Read the model definition and answer for the solid it produces. Units are mm, in the model's axes. A direction names the side the tool comes from. Coordinates: 2 decimals unless noted, no trailing zeros. Order: outer loops, then holes, each group sorted by start corner. A loop starts at its lowest first (then second) coordinate and runs counter-clockwise, first axis right, second up. Notation, with made-up numbers: (46, -19.75) -> (96, -19.75) arc R30 ccw to (96, 13.25) -> close; hole circle Ø9 at (66.5, 72). An arc over 180 degrees is marked (long way). Use CSV: the item, a comma, the result in double quotes.
```python
from build123d import *

# Parameters (mm, degrees)
SKETCH1_R           = 2.75
SKETCH1_R_2         = 1.475
BOSS_EXTRUDE1_DEPTH = 31.95
BOSS_EXTRUDE2_START = -31.95
BOSS_EXTRUDE2_DEPTH = 31.95
SKETCH3_R           = 1.475
BOSS_EXTRUDE3_DEPTH = 31.95
SKETCH4_R           = 1.475
CUT_EXTRUDE1_DEPTH  = 10
CUT_EXTRUDE2_START  = -10
SKETCH5_R           = 1.475
CUT_EXTRUDE2_DEPTH  = 10


with BuildPart() as part:
    # Sketch1 → Boss-Extrude1 (new body)
    with BuildSketch(Plane.XY):
        Circle(SKETCH1_R)
        Circle(SKETCH1_R_2, mode=Mode.SUBTRACT)
    extrude(amount=BOSS_EXTRUDE1_DEPTH)

    # Sketch2 → Boss-Extrude2 (add)
    with BuildSketch(Plane.XY.offset(31.95).offset(BOSS_EXTRUDE2_START)):
        with BuildLine():
            ThreePointArc((0, -2.75), (-1.944543648, -1.944543648), (-2.75, 0))
            Line((-2.75, 0), (-2.75, -2.75))
            Line((-2.75, -2.75), (0, -2.75))
        make_face()
        with BuildLine():
            Line((2.75, -2.75), (2.75, 0))
            ThreePointArc((2.75, 0), (1.944543648, -1.944543648), (0, -2.75))
            Line((0, -2.75), (2.75, -2.75))
        make_face()
    extrude(amount=BOSS_EXTRUDE2_DEPTH)

    # Sketch3 → Boss-Extrude3 (add)
    with BuildSketch(Plane(origin=(0, 0, 0), x_dir=(-1, 0, 0), z_dir=(0, 0, -1))):
        Circle(SKETCH3_R)
    extrude(amount=-BOSS_EXTRUDE3_DEPTH)

    # Sketch4 → Cut-Extrude1 (cut)
    with BuildSketch(Plane(origin=(0, 0, 0), x_dir=(-1, 0, 0), z_dir=(0, 0, -1))):
        Circle(SKETCH4_R)
    extrude(amount=-CUT_EXTRUDE1_DEPTH, mode=Mode.SUBTRACT)

    # Sketch5 → Cut-Extrude2 (cut)
    with BuildSketch(Plane.XY.offset(31.95).offset(CUT_EXTRUDE2_START)):
        with Locations(Location((0, 0, 0), (0, 0, 180))):
            Circle(SKETCH5_R)
    extrude(amount=CUT_EXTRUDE2_DEPTH, mode=Mode.SUBTRACT)


solid = part.part
```
Item 1: Find section A-A, the plane z = 8.5. Give the vertices of the cut face in (x, y) (3 decimals), then the cut area to 3 significant figures.
Return value:
outline,"(-2.75, -2.75) -> (2.75, -2.75) -> (2.75, 0) arc R2.75 ccw to (-2.75, 0) -> close; hole circle Ø2.95 at (0, 0)"
area,"20.2 mm^2"
Item 2: Straight lines are drawn through the part: line 1 along Y through (x, z) = (0, 29.75) (3 decimals); line 2 along Y through (x, z) = (-0.9, 24); line 3 along Z through (x, y) = (0.5, -0.3). For each, find the intervals that lie inside material, in ascending order.
Return value:
line 1,"y = -2.75 to -1.475, 1.475 to 2.75"
line 2,"y = -2.75 to -1.17, 1.17 to 2.6"
line 3,"z = 10 to 21.95"
Item 3: Find section D-D, the plane z = 15. Give the vertices of the cut face in (x, y), then the cut area to 3 significant figures.
Return value:
outline,"(-2.75, -2.75) -> (2.75, -2.75) -> (2.75, 0) arc R2.75 ccw to (-2.75, 0) -> close"
area,"27.0 mm^2"
Item 4: Find section B-B, the plane x = 0. Give the vertices of the cut face in (y, z) (3 decimals).
Return value:
outline,"(-2.75, 0) -> (-1.475, 0) -> (-1.475, 10) -> (1.475, 10) -> (1.475, 0) -> (2.75, 0) -> (2.75, 31.95) -> (1.475, 31.95) -> (1.475, 21.95) -> (-1.475, 21.95) -> (-1.475, 31.95) -> (-2.75, 31.95) -> close"
Item 5: The mould has two halves that part along Y. Classify faces 1 (the cylindrical face through (0.06, 2.75, 15.75)), 2 (the flat face through (-2.75, -1, 16)), 3 (the flat face through (0, -2.75, 16)), 4 (the flat face through (0, 0, 10)): +Y half, -Y half, draft (parallel to the pull), parting line (faces both ways), or undercut.
Return value:
face 1,"+Y half"
face 2,"draft"
face 3,"-Y half"
face 4,"undercut"
Item 6: A tool of negligible diameter and unlimited length cuts with its end or side. For faces 5 (the cylindrical face through (1.474, -0.065, 26.88)), 6 (the cylindrical face through (1.474, 0.065, 4.93)), 7 (the flat face through (-1.2, -1.2, 0)), from which of +Z, -Z, +X, -X, +Y, -Y can it reach the whole face along a straight path? Write none if from no direction.
Return value:
face 5,"+Z"
face 6,"-Z"
face 7,"-Z, +X, -X, +Y, -Y"
Item 7: Each of these flat-tipped pins is pushed along its axis until it touches: P1, Ø2.5, axis at x = 0, y = 0, coming from the -Z side; P2, Ø1.8, axis at x = 0, y = 0, coming from the +Z side. Where does it stop, or does it pass through?
Return value:
P1,"stops at z = 10"
P2,"stops at z = 21.95"
Item 8: Find section C-C, the plane y = -1.2. Give the vertices of the cut face in (x, z).
Return value:
outline,"(-2.75, 0) -> (-0.86, 0) -> (-0.86, 10) -> (0.86, 10) -> (0.86, 0) -> (2.75, 0) -> (2.75, 31.95) -> (0.86, 31.95) -> (0.86, 21.95) -> (-0.86, 21.95) -> (-0.86, 31.95) -> (-2.75, 31.95) -> close"
